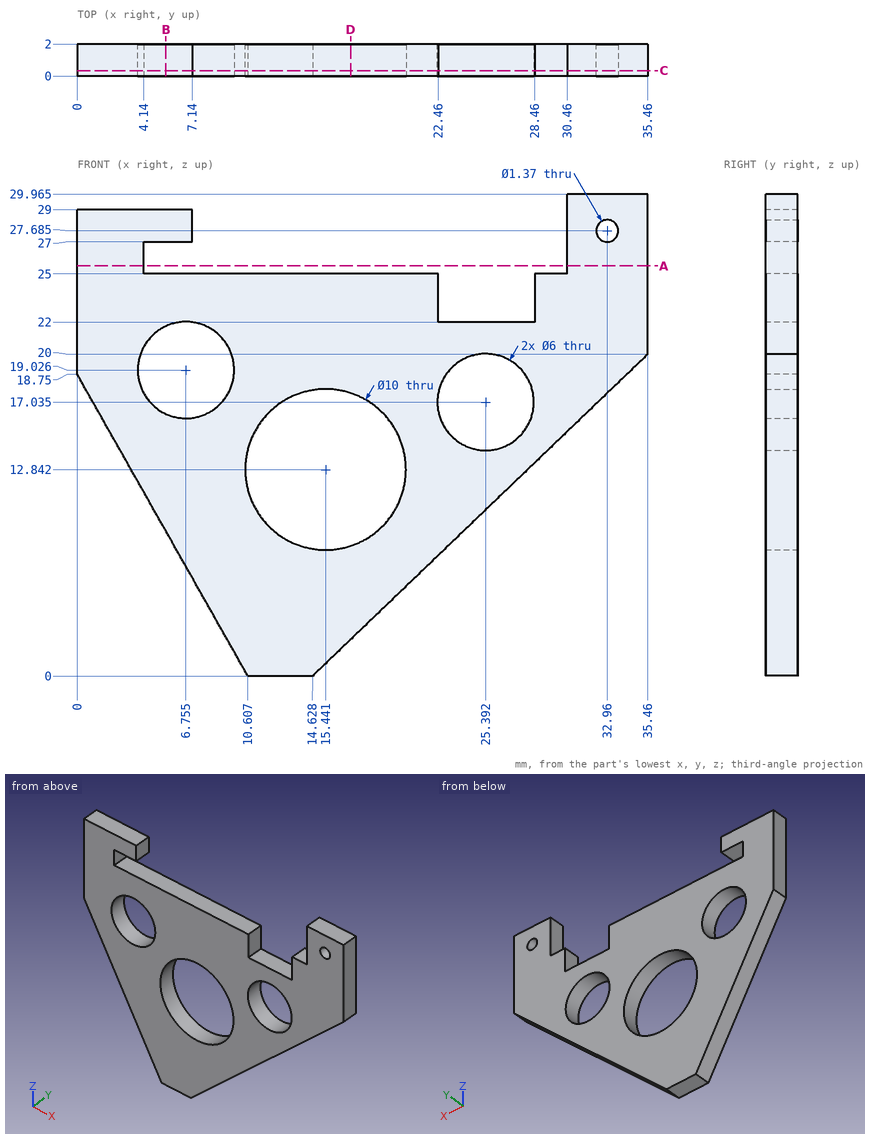
Design review of the part shown in the three views and the two pictorial views. Dimensions are in mm from the part's minimum x, y and z. Give positions to 0.01 mm unless a question says otherwise; leave off trailing zeros. Write each loop counter-clockwise with the first axis right and the second up, starting at its lowest first coordinate (ties: lowest second). Pieces come first, ordered by that corner, then holes. Notation, with made-up numbers: M -28.75,39.25 L 12.25,39.25 A5 ccw 12.25,47.25 Z; hole C 30,51.25 d10. An arc over 180 degrees is marked long. One line per question, with ' | ' between items. Start each with the question number.
Item 1: For pin 1 (1 mm diameter, centred on x = 4.5, y = 0.5, fed in from +Z); pin 2 (0.6 mm diameter, centred on x = 29, y = 0.5, fed in from +Z); pin 3 (1 mm diameter, centred on x = 5.5, y = 1, fed in from -Z) (1 decimal), all flat-tipped, find the tip position at first contact; note any pin that passes through.
Item 2: We need section A-A on z = 25.5. Write out the cut boundary in (x, y).
Item 3: We need section C-C on y = 0.35. Give the number of separate pieces and of enclosed holes in the cut face.
Item 4: We need section D-D on x = 17. Write out the cut boundary in (y, z).
Item 5: We need section B-B on x = 5.5. Write out the cut boundary in (y, z).
Item 6: Wall thickness on line 1 (X direction, y = 0.45, z = 22.5); line 2 (Z direction, x = 24, y = 1.85) (1 decimal); line 3 (Z direction, x = 11, y = 0.35) (1 decimal): over which ranges is each line inside the solid? List them lowest first. Write a range as from..to.
Results found:
1) pin 1: stops at z = 29 | pin 2: stops at z = 25 | pin 3: stops at z = 8.1
2) outline: M 0,0 L 4.14,0 L 4.14,2 L 0,2 Z; M 30.46,0 L 35.46,0 L 35.46,2 L 30.46,2 Z
3) separate pieces: 1 | enclosed holes: 4
4) outline: M 0,2.28 L 2,2.28 L 2,8.09 L 0,8.09 Z; M 0,17.59 L 2,17.59 L 2,25 L 0,25 Z
5) outline: M 0,9.03 L 2,9.03 L 2,16.3 L 0,16.3 Z; M 0,21.75 L 2,21.75 L 2,25 L 0,25 Z; M 0,27 L 2,27 L 2,29 L 0,29 Z
6) line 1: x = 0..22.46, 28.46..35.46 | line 2: z = 9..14.4, 19.7..22 | line 3: z = 0..10.5, 15.1..25
